Here's how the part is built. I have some questions about the finished solid (model axes, mm). A direction names the side the tool comes from. Round coordinates to 2 decimals unless told otherwise and drop trailing zeros. Write each loop counter-clockwise with the first axis right and the second up, starting at its lowest first coordinate (ties: lowest second). Pieces come first, ordered by that corner, then holes. Notation, with made-up numbers: (-16.5, 35.25) -> (-7.5, 35.25) arc R15 cw to (-7.5, 55.25) -> close; hole circle Ø1 at (-1, 81.25). An arc over 180 degrees is marked (long way). Answer in a Markdown table with one row per item.
from build123d import *

# Parameters (mm, degrees)
F0_R      = 15.875
F1_DEPTH  = 31.75
F3_R      = 6.35
F4_DEPTH  = 44.45
F6_R      = 4.445
F7_DEPTH  = 76.2
F9_R      = 4.445
F10_DEPTH = 76.2


with BuildPart() as f1:
    # F0 (on Top) → F1 (new body)
    with BuildSketch(Plane.XY):
        Circle(F0_R)
    extrude(amount=-F1_DEPTH)

    # F3 (on offset) → F4 (join)
    with BuildSketch(Plane.XY.offset(-76.2)):
        Circle(F3_R)
    extrude(amount=F4_DEPTH)

    # F6 (on offset) → F7 (join)
    with BuildSketch(Plane.YZ.offset(76.2)):
        with Locations((0, -15.875)):
            Circle(F6_R)
    extrude(amount=-F7_DEPTH)

    # F9 (on offset) → F10 (join)
    with BuildSketch(Plane.YZ.offset(-76.2)):
        with Locations((0, -15.875)):
            Circle(F9_R)
    extrude(amount=F10_DEPTH)

    # F11 (on Front) → F12 (revolve)
    with BuildSketch(Plane.XZ):
        with BuildLine():
            Line((-116.347869, -15.875), (-76.2, -15.875))
            Line((-76.2, -15.875), (-76.2, -11.43))
            ThreePointArc((-76.2, -11.43), (-98.75608, 8.766592), (-116.347869, -15.875))
        make_face()
    revolve(axis=Axis((-68.523894, 0, -15.875), (-1, 0, 0)))

    # F11 (on Front) → F13 (revolve)
    with BuildSketch(Plane.XZ):
        with BuildLine():
            Line((76.2, -11.43), (76.2, -15.875))
            Line((76.2, -15.875), (116.347869, -15.875))
            ThreePointArc((116.347869, -15.875), (98.75608, 8.766592), (76.2, -11.43))
        make_face()
    revolve(axis=Axis((-68.523894, 0, -15.875), (-1, 0, 0)))


solid = f1.part
1) We'd pull the mould along X, two halves only. Please class faces 1 (the face through (-46.15, -0.58, -11.47)), 2 (the face through (0, 0, -76.2)): +X half, -X half, draft (parallel to the pull), parting line (faces both ways), or undercut.
Response:
| item | result |
|---|---|
| face 1 | undercut |
| face 2 | draft |
2) I want a section at B-B, the plane z = -45. List the corners of the cut face in (x, y) for me, and give its area (3 significant figures).
Response:
| item | result |
|---|---|
| outline | circle Ø12.7 at (0, 0) |
| area | 127 mm^2 |
3) I want a section at D-D, the plane x = -41. List the corners of the cut face in (y, z) for me (3 decimals).
Response:
| item | result |
|---|---|
| outline | circle Ø8.89 at (0, -15.875) |
4) I need wall thicknesses on line 1 (X direction, y = -8.5, z = -7.5); line 2 (X direction, y = -14, z = -26); line 3 (X direction, y = 15, z = 0.5). Which ranges of each line are inside material? Lowest first, please. Write a range as [from, to].
Response:
| item | result |
|---|---|
| line 1 | x = [-115.41, -77.63], [-13.41, 13.41], [77.63, 115.41] |
| line 2 | x = [-112.28, -80.76], [-7.48, 7.48], [80.76, 112.28] |
| line 3 | x = [-106.39, -86.65], [86.65, 106.39] |
5) Which directions (+Z, -Z, +X, -X, +Y, -Y) give clear straight access to the entire face, cutting with the end or side of a thin tool? Please do faces 3 (the face through (0, 0, 0)), 4 (the face through (46.15, -0.58, -11.47)), 5 (the face through (-1.38, -6.2, -54.29)).
Response:
| item | result |
|---|---|
| face 3 | +Z, +Y, -Y |
| face 4 | none |
| face 5 | -Z |
6) For pin 1 (4 mm diameter, centred on y = -9, z = -53.5, fed in from -X); pin 2 (16 mm diameter, centred on x = -5, y = -3, fed in from +Z); pin 3 (3 mm diameter, centred on x = 87.5, y = 10.5, fed in from +Z); pin 4 (4 mm diameter, centred on y = -11, z = -10, fed in from +X), each with a flat end and sliding along its axis, tell me the tip position at first contact or that it passes through.
Response:
| item | result |
|---|---|
| pin 1 | passes through |
| pin 2 | stops at z = 0 |
| pin 3 | stops at z = 5.25 |
| pin 4 | stops at x = 115.93 |
7) I want a section at C-C, the plane y = -10.5. Count the separate pieces of the cut face and the enclosed holes in it, and give its area (3 significant figures).
Response:
| item | result |
|---|---|
| separate pieces | 3 |
| enclosed holes | 0 |
| area | 3,540 mm^2 |
8) I want a section at A-A, the plane x = 0. List the corners of the cut face in (y, z) for me (3 decimals).
Response:
| item | result |
|---|---|
| outline | (-15.875, -31.75) -> (-6.35, -31.75) -> (-6.35, -76.2) -> (6.35, -76.2) -> (6.35, -31.75) -> (15.875, -31.75) -> (15.875, 0) -> (-15.875, 0) -> close |
